```python
from build123d import *

# Parameters (mm, degrees)
SKETCH_1_R          = 28
SKETCH_1_R_2        = 7.5
EXTRUDE_1_DEPTH     = 10
SKETCH_2_R          = 17.5
SKETCH_2_R_2        = 7.5
EXTRUDE_2_DEPTH     = 27
SKETCH_3_R          = 2.75
CUT_EXTRUDE_1_DEPTH = 27


with BuildPart() as part:
    # 草图1 → 凸台-拉伸1 (new body)
    with BuildSketch(Plane(origin=(0, 0, 0), x_dir=(1, 0, 0), z_dir=(0, 1, 0))):
        Circle(SKETCH_1_R)
        Circle(SKETCH_1_R_2, mode=Mode.SUBTRACT)
    extrude(amount=EXTRUDE_1_DEPTH)

    # 草图2 → 凸台-拉伸2 (add)
    with BuildSketch(Plane(origin=(0, 10, 0), x_dir=(1, 0, 0), z_dir=(0, 1, 0))):
        Circle(SKETCH_2_R)
        Circle(SKETCH_2_R_2, mode=Mode.SUBTRACT)
    extrude(amount=EXTRUDE_2_DEPTH)

    # 草图3 → 切除-拉伸1 (cut)
    with BuildSketch(Plane(origin=(0, 10, 0), x_dir=(1, 0, 0), z_dir=(0, 1, 0))):
        with Locations((0, 23)):
            Circle(SKETCH_3_R)
        with Locations((23, 0)):
            Circle(SKETCH_3_R)
        with Locations((0, -23)):
            Circle(SKETCH_3_R)
        with Locations((-23, 0)):
            Circle(SKETCH_3_R)
    extrude(amount=-CUT_EXTRUDE_1_DEPTH, mode=Mode.SUBTRACT)


solid = part.part
```
Geometry: final body of the model. Coordinates: model frame, mm. A direction names the side the tool comes from. Round coordinates to 2 decimals unless told otherwise and drop trailing zeros. Loops run counter-clockwise (first coordinate to the right, second up) from the corner with the lowest first, then second, coordinate; pieces in that order, holes last.
Item 1: Mould query, pull axis Z, two halves, no side actions, for faces 1 (the cylindrical face through (-0.358, 5.07, 20.273)), 2 (the cylindrical face through (25.865, 4.93, 10.724)), 3 (the flat face through (6, 0, 6)), 4 (the cylindrical face through (20.253, 5.07, -0.121)). Classes: released by +Z, released by -Z, zero draft, split by the parting line, or undercut.
Checked values:
face 1: undercut
face 2: split by the parting line
face 3: zero draft
face 4: undercut
Item 2: Reachability of faces 5 (the flat face through (0, 37, 8)), 6 (the flat face through (-13, 10, 12)) from +Z, -Z, +X, -X, +Y, -Y: full face, straight path, thin tool, end or side. Return the list, or none.
Checked values:
face 5: +Z, -Z, +X, -X, +Y
face 6: +Y
Item 3: Contact query for flat-ended pins moving along their axis: P1, Ø10, axis at y = 6, z = -11, coming from the +X side; P2, Ø3.5, axis at x = 23, z = 0, coming from the +Y side; P3, Ø1.5, axis at x = -21.5, z = -7, coming from the +Y side; P4, Ø10, axis at x = -16, y = 7, coming from the -Z side. Output: stop coordinate, or through.
Checked values:
P1: stops at x = 27.35
P2: passes through
P3: stops at y = 10
P4: stops at z = -25.75
Item 4: Section A-A, the plane x = 0. Output: boundary loops of the cut face in (y, z), plus the area to 3 significant figures.
Checked values:
outline: (0, -28) - (10, -28) - (10, -25.75) - (0, -25.75) - close; (0, -20.25) - (10, -20.25) - (10, -17.5) - (37, -17.5) - (37, -7.5) - (0, -7.5) - close; (0, 7.5) - (37, 7.5) - (37, 17.5) - (10, 17.5) - (10, 20.25) - (0, 20.25) - close; (0, 25.75) - (10, 25.75) - (10, 28) - (0, 28) - close
area: 840 mm2
Item 5: Section C-C, the plane y = 8. Output: boundary loops of the cut face in (x, z), plus the area to 3 significant figures.
Checked values:
outline: circle Ø56 at (0, 0); hole circle Ø5.5 at (-23, 0); hole circle Ø15 at (0, 0); hole circle Ø5.5 at (0, -23); hole circle Ø5.5 at (0, 23); hole circle Ø5.5 at (23, 0)
area: 2,190 mm2
Item 6: Line query: L1, parallel to X at y = 2, z = 0; L2, parallel to Z at x = -0.5, y = 5; L3, parallel to Z at x = -0.5, y = 16.5. Output: solid intervals per line, ascending.
Checked values:
L1: x = -28 to -25.75, -20.25 to -7.5, 7.5 to 20.25, 25.75 to 28
L2: z = -28 to -25.7, -20.3 to -7.48, 7.48 to 20.3, 25.7 to 28
L3: z = -17.49 to -7.48, 7.48 to 17.49
Item 7: Section B-B, the plane z = 4.5. Output: boundary loops of the cut face in (x, y), plus the area to 3 significant figures.
Checked values:
outline: (-27.64, 0) - (-6, 0) - (-6, 37) - (-16.91, 37) - (-16.91, 10) - (-27.64, 10) - close; (6, 0) - (27.64, 0) - (27.64, 10) - (16.91, 10) - (16.91, 37) - (6, 37) - close
area: 1,020 mm2
Item 8: Section D-D, the plane x = -23. Output: boundary loops of the cut face in (y, z), plus the area to 3 significant figures.
Checked values:
outline: (0, -15.97) - (10, -15.97) - (10, -2.75) - (0, -2.75) - close; (0, 2.75) - (10, 2.75) - (10, 15.97) - (0, 15.97) - close
area: 264 mm2
